```python
from build123d import *

# Parameters (mm, degrees)
BOSS_EXTRUDE2_DEPTH = 4.75


with BuildPart() as part:
    # Sketch1 → Boss-Extrude2 (new body)
    with BuildSketch(Plane(origin=(0, 0, 0), x_dir=(1, 0, 0), z_dir=(0, 1, 0))):
        Polygon((100, 60), (-75, 60), (-110, 25), (-130, 25), (-130, -25), (-110, -25), (-75, -60), (100, -60), (135, -25), (155, -25), (155, 25), (135, 25), align=None)
        with BuildLine():
            ThreePointArc((-0.096105451, 15.808688779), (-0.437294407, 15.700808335), (-0.778483364, 15.808688779))
            Line((-0.778483364, 15.808688779), (-0.096105451, 15.808688779))
        make_face(mode=Mode.SUBTRACT)
    extrude(amount=BOSS_EXTRUDE2_DEPTH)


solid = part.part
```
Model file for the job. Use its own axes, mm. A direction names the side the tool comes from. Coordinates: 2 decimals unless noted, no trailing zeros. Order: outer loops, then holes, each group sorted by start corner. A loop starts at its lowest first (then second) coordinate and runs counter-clockwise, first axis right, second up. Notation, with made-up numbers: (89, -18) - (121, -18) arc R26 cw to (121, 14) - close; hole circle Ø3 at (-16.75, 71.25). An arc over 180 degrees is marked (long way). Return JSON: item names as keys, results as strings. Group by question number.
1) Flat gauge pins, fed straight in: P1, Ø1.4, axis at x = 141.5, y = 2.5, coming from the +Z side; P2, Ø1.4, axis at x = 142, y = 3.5, coming from the -Z side; P3, Ø1.5, axis at x = 114.5, z = -40, coming from the -Y side. Where does each tip first touch, or does it go through?
2) Tool access for faces 1 (the flat face through (145, 2, 25)), 2 (the flat face through (-120, 2, -25)), 3 (the flat face through (145, 2, -25)): list every direction of +Z, -Z, +X, -X, +Y, -Y with a clear straight run to the whole face (end or side of a thin tool).
3) Saw through at B-B, the plane x = -101. Write the cut outline in (y, z).
4) Probe line 1 (Z direction, x = 108, y = 4.4); line 2 (X direction, y = 4.4, z = -51); line 3 (X direction, y = 4, z = -45). List the from-to ranges inside material, lowest first. Write a range as from..to.
5) Saw through at C-C, the plane z = -42.5. Write the cut outline in (x, y).
6) Saw through at A-A, the plane y = 2.3. Write the cut outline in (x, z).
Values found:
{
 "1": {"P1": "stops at z = 25", "P2": "stops at z = -25", "P3": "stops at y = 0"},
 "2": {"face 1": "+Z, +X, +Y, -Y", "face 2": "-Z, -X, +Y, -Y", "face 3": "-Z, +X, +Y, -Y"},
 "3": {"outline": "(0, -34) - (4.75, -34) - (4.75, 34) - (0, 34) - close"},
 "4": {"line 1": "z = -52..52", "line 2": "x = -84..109", "line 3": "x = -90..115"},
 "5": {"outline": "(-92.5, 0) - (117.5, 0) - (117.5, 4.75) - (-92.5, 4.75) - close"},
 "6": {"outline": "(-130, -25) - (-110, -25) - (-75, -60) - (100, -60) - (135, -25) - (155, -25) - (155, 25) - (135, 25) - (100, 60) - (-75, 60) - (-110, 25) - (-130, 25) - close; hole (-0.78, -15.81) - (-0.1, -15.81) arc R0.59 ccw to start"}
}
